Can you work these out from the drawing? Everything is in mm from the part's minimum corner. A direction names the side the tool comes from. Round coordinates to 2 decimals unless told otherwise and drop trailing zeros. Order: outer loops, then holes, each group sorted by start corner. A loop starts at its lowest first (then second) coordinate and runs counter-clockwise, first axis right, second up. Notation, with made-up numbers: M 42,2 L 61,2 A9 ccw 61,18 Z; hole C 68.5,-36.75 d2. An arc over 180 degrees is marked long. Write each question's results on one line, items separated by ' | '. Start each with the question number.
1. Suppose I cut it at B-B on y = 47. Write out the boundary of the cut face in (x, z).
2. For the marked faces 5, 6 and 7, which set-ups out of +Z, -Z, +X, -X, +Y, -Y let a thin tool reach every point of the face, with its end or its side?
3. We'd pull the mould along X, two halves only. Please class the marked faces 1, 2, 3 and 4: released by +X, released by -X, zero draft, split by the parting line, or undercut.
4. I'm going to push flat-ended pins straight in: pin 1 (12 mm diameter, centred on y = 20.5, z = 10.5, fed in from -X); pin 2 (12 mm diameter, centred on x = 17.5, y = 35, fed in from -Z); pin 3 (4 mm diameter, centred on x = 2, y = 45, fed in from -Z); pin 4 (1.8 mm diameter, centred on x = 2, z = 3, fed in from +Y). Where does each tip first touch, or does it pass through?
5. Suppose I cut it at A-A on x = 22.5. Write out the boundary of the cut face in (y, z).
6. Suppose I cut it at C-C on x = 39. Write out the boundary of the cut face in (y, z), and give its area (3 significant figures).
7. Please list where these lines run through material, in increasing order: L1, parallel to X at y = 47.5, z = 38; L2, parallel to Y at x = 27, z = 34; L3, parallel to Z at x = 13, y = 25.5.
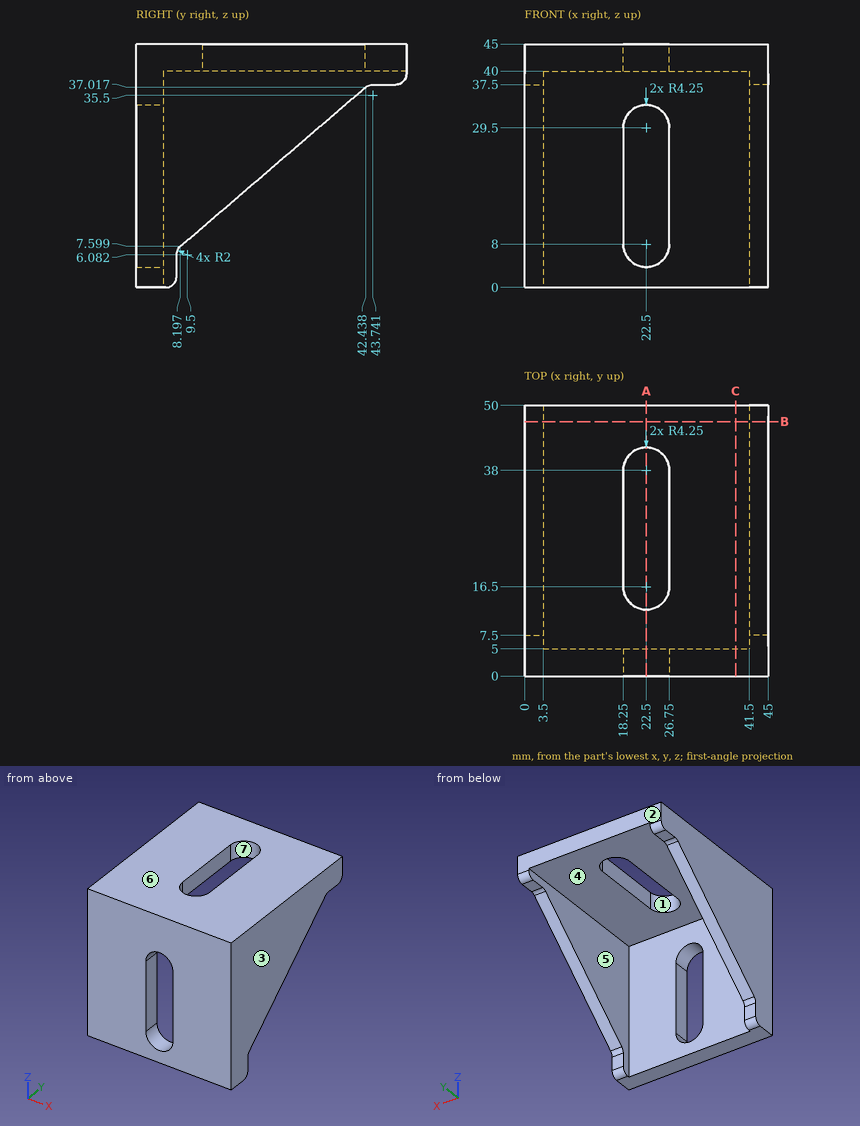
Filled sheet:
1) outline: M 0,37.5 L 3.5,37.5 L 3.5,40 L 41.5,40 L 41.5,37.5 L 45,37.5 L 45,45 L 0,45 Z
2) face 5: -Z, +Y | face 6: +Z, +X, -X, +Y, -Y | face 7: +Z, -Z
3) face 1: undercut | face 2: zero draft | face 3: released by +X | face 4: undercut
4) pin 1: stops at x = 0 | pin 2: stops at z = 40 | pin 3: stops at z = 37.36 | pin 4: stops at y = 7.5
5) outline: M 0,0 L 5,0 L 5,3.75 L 0,3.75 Z; M 0,33.75 L 5,33.75 L 5,40 L 12.25,40 L 12.25,45 L 0,45 Z; M 42.25,40 L 50,40 L 50,45 L 42.25,45 Z
6) outline: M 0,0 L 5,0 L 5,40 L 50,40 L 50,45 L 0,45 Z | area: 450 mm^2
7) L1: x = 0 to 3.5, 41.5 to 45 | L2: y = 0 to 5 | L3: z = 40 to 45
